Part model, mm, in its own coordinate system. Face numbers are marked on the shaded views. A direction names the side the tool comes from. Give positions to 0.01 mm unless a question says otherwise; leave off trailing zeros. Order: outer loops, then holes, each group sorted by start corner. A loop starts at its lowest first (then second) coordinate and runs counter-clockwise, first axis right, second up. Notation, with made-up numbers: (50, 82.25) - (79, 82.25) arc R10 ccw to (79, 95.25) - close; hole circle Ø2 at (-3.75, 48.5). An arc over 180 degrees is marked (long way). Use one line per item in the form item = value. Start each with the question number.
1. Drill centre lines: line 1 (X direction, y = 15.5, z = 9) (3 decimals); line 2 (X direction, y = 2.75, z = 28); line 3 (Z direction, x = -22, y = 15). Where is each one in solid material? Low to high.
2. Pull direction Z, two halves, no side cores. Call the marked faces 1, 2 and 3: +Z half, -Z half, draft (parallel to the pull), parting line (faces both ways), or undercut.
3. Band-saw the part on A-A, the plane x = 12.7. List the corners of the cut face in (y, z) (3 decimals).
4. Band-saw the part on D-D, the plane x = -11. List the corners of the cut face in (y, z).
5. Tool access for the marked faces 4, 5, 6, 7 and 8: list every direction of +Z, -Z, +X, -X, +Y, -Y with a clear straight run to the whole face (end or side of a thin tool).
6. Band-saw the part on C-C, the plane y = 17.5. List the corners of the cut face in (x, z) (3 decimals), plus the area to 3 significant figures.
7. Band-saw the part on B-B, the plane z = 0. List the corners of the cut face in (x, y) (3 decimals).
8. Pin check, flat tips, straight feed: P1, Ø1, axis at x = 23.5, y = 16.5, coming from the -Z side; P2, Ø12, axis at x = 21.5, y = 16.5, coming from the +Z side; P3, Ø6.5, axis at x = 14, z = -29.5, coming from the +Y side (3 decimals). Stop position of each tip, or through.
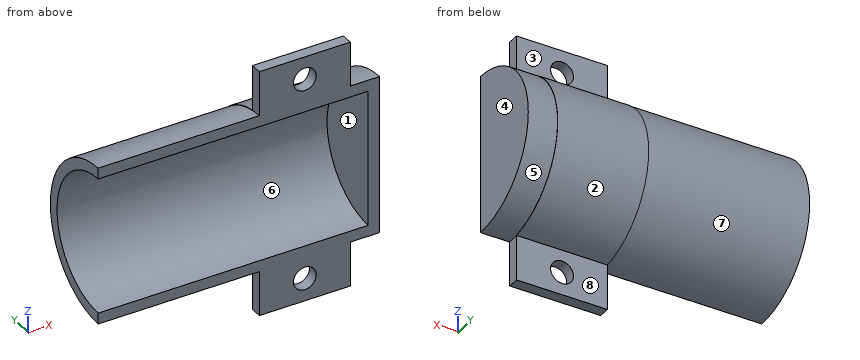
from build123d import *

# Parameters (mm, degrees)
BOSS_EXTRUDE1_DEPTH = 25.4
SKETCH2_R           = 3.175
CUT_EXTRUDE1_DEPTH  = 25.4
SKETCH3_R           = 3.175
CUT_EXTRUDE2_DEPTH  = 25.4
BOSS_EXTRUDE2_DEPTH = 5
BOSS_EXTRUDE3_DEPTH = 3.175
BOSS_EXTRUDE4_DEPTH = 45


with BuildPart() as part:
    # Sketch1 → Boss-Extrude1 (new body)
    with BuildSketch(Plane(origin=(0, 0, 0), x_dir=(0, 0, -1), z_dir=(1, 0, 0))):
        with BuildLine():
            Line((19, 0), (34.546525921, 0))
            Line((34.546525921, 0), (34.546525921, 3.175))
            Line((34.546525921, 3.175), (21.946525921, 3.175))
            ThreePointArc((21.946525921, 3.175), (0, 22.175), (-21.946525921, 3.175))
            Line((-21.946525921, 3.175), (-34.546525921, 3.175))
            Line((-34.546525921, 3.175), (-34.546525921, 0))
            Line((-34.546525921, 0), (-19, 0))
            ThreePointArc((-19, 0), (0, 19), (19, 0))
        make_face()
    extrude(amount=BOSS_EXTRUDE1_DEPTH)

    # Sketch2 → Cut-Extrude1 (cut)
    with BuildSketch(Plane(origin=(0, 3.175, 0), x_dir=(1, 0, 0), z_dir=(0, 1, 0))):
        with Locations(Location((12.7, -28.196525921, 0), (0, 0, 270))):
            Circle(SKETCH2_R)
    extrude(amount=-CUT_EXTRUDE1_DEPTH, mode=Mode.SUBTRACT)

    # Sketch3 → Cut-Extrude2 (cut)
    with BuildSketch(Plane(origin=(0, 3.175, 0), x_dir=(1, 0, 0), z_dir=(0, 1, 0))):
        with Locations(Location((12.7, 28.196525921, 0), (0, 0, 270))):
            Circle(SKETCH3_R)
    extrude(amount=-CUT_EXTRUDE2_DEPTH, mode=Mode.SUBTRACT)

    # Sketch4 → Boss-Extrude2 (add)
    with BuildSketch(Plane(origin=(25.4, 0, 0), x_dir=(0, 0, -1), z_dir=(1, 0, 0))):
        with BuildLine():
            Line((-22.104651978, 0), (-19, 0))
            ThreePointArc((-19, 0), (0, 19), (19, 0))
            Line((19, 0), (22.104651978, 0))
            ThreePointArc((22.104651978, 0), (0, 22.104651978), (-22.104651978, 0))
        make_face()
    extrude(amount=BOSS_EXTRUDE2_DEPTH)

    # Sketch5 → Boss-Extrude3 (add)
    with BuildSketch(Plane(origin=(30.4, 0, 0), x_dir=(0, 0, -1), z_dir=(1, 0, 0))):
        with BuildLine():
            ThreePointArc((22.104651978, 0), (0, 22.104651978), (-22.104651978, 0))
            Line((-22.104651978, 0), (22.104651978, 0))
        make_face()
    extrude(amount=BOSS_EXTRUDE3_DEPTH)

    # Sketch6 → Boss-Extrude4 (add)
    with BuildSketch(Plane.ZY):
        with BuildLine():
            ThreePointArc((-19, 0), (0, 19), (19, 0))
            Line((19, 0), (21.402036048, 0))
            Line((21.402036048, 0), (22.079689898, 0))
            ThreePointArc((22.079689898, 0), (0, 22.079689898), (-22.079689898, 0))
            Line((-22.079689898, 0), (-19, 0))
        make_face()
    extrude(amount=BOSS_EXTRUDE4_DEPTH)


solid = part.part
From the geometry:
q1.line_1 = 30.4 to 33.575
q1.line_2 = 0 to 9.53, 15.87 to 25.4
q1.line_3 = -16.2 to -11.66, 11.66 to 16.2
q2.face_1 = undercut
q2.face_2 = parting line
q2.face_3 = draft
q3.outline = (0, -34.547) - (3.175, -34.547) - (3.175, -31.372) - (0, -31.372) - close; (0, -25.022) - (3.175, -25.022) - (3.175, -21.947) arc R22.175 ccw to (3.175, 21.947) - (3.175, 25.022) - (0, 25.022) - (0, 19) arc R19 cw to (0, -19) - close; (0, 31.372) - (3.175, 31.372) - (3.175, 34.547) - (0, 34.547) - close
q4.outline = (0, -22.08) arc R22.08 ccw to (0, 22.08) - (0, 19) arc R19 cw to (0, -19) - close
q5.face_4 = +Z, -Z, +X, +Y, -Y
q5.face_5 = +X, +Y
q5.face_6 = -X, -Y
q5.face_7 = -X, +Y
q5.face_8 = -Z, +X, -X, +Y
q6.outline = (-45, -13.463) - (0, -13.463) - (0, -13.619) - (25.4, -13.619) - (25.4, -13.504) - (33.575, -13.504) - (33.575, 13.504) - (25.4, 13.504) - (25.4, 13.619) - (0, 13.619) - (0, 13.463) - (-45, 13.463) - (-45, 7.399) - (30.4, 7.399) - (30.4, -7.399) - (-45, -7.399) - close
q6.area = 1,010 mm²
q7.outline = (-45, 19) - (30.4, 19) - (30.4, 0) - (33.575, 0) - (33.575, 22.105) - (25.4, 22.105) - (25.4, 22.175) - (0, 22.175) - (0, 22.08) - (-45, 22.08) - close
q8.P1 = -15.35
q8.P2 = 19.53
q8.P3 = 3.175
